Geometry: final body of the model. Coordinates: model frame, mm. A direction names the side the tool comes from. Coordinates: 2 decimals unless noted, no trailing zeros. Order: outer loops, then holes, each group sorted by start corner. A loop starts at its lowest first (then second) coordinate and runs counter-clockwise, first axis right, second up. Notation, with made-up numbers: M 71.25,-22.5 L 75.25,-22.5 A27 ccw 75.25,2.5 Z; hole C 10,89.5 d2. An arc over 180 degrees is marked long. Use CSV: the item, a comma, the result in double quotes. Start each with the question number.
Q1. Section query B-B, the plane y = 0.5. Output: boundary loops of the cut face in (x, z).
Q2. First-contact query: P1, Ø0.5, axis at y = -2.5, z = 1.5, coming from the -X side; P2, Ø2.5, axis at y = -11, z = 3, coming from the -X side; P3, Ø5, axis at x = -29, y = -5, coming from the +Z side. Flat tips, straight axial feed; report the tip coordinate or a pass-through.
Q3. Ray query, probe 1 along Z at (x, y) = (-27, -16.75); probe 2 along X at (y, z) = (2.25, 1.1); probe 3 along X at (y, z) = (-11, 2.65). Return the intervals inside material, ascending.
Q4. Section query A-A, the plane z = 0.4. Output: boundary loops of the cut face in (x, y), and give its area (3 significant figures).
Q5. Section query C-C, the plane x = -43.25. Output: boundary loops of the cut face in (y, z).
Q6. Section query D-D, the plane z = 3.25. Output: boundary loops of the cut face in (x, y).
Q7. Access query for faces 1 (the face through (-31.029, 1.2, 1.5)), 2 (the face through (-33.847, -3.4, 1.5)), 3 (the face through (-38.809, -9, 2)). Directions: +Z, -Z, +X, -X, +Y, -Y. A direction counts if a zero-diameter tool reaches every point of the face in a straight line with its end or side. Return the directions, or none.
Q8. Mould query, pull axis Y, two halves, no side actions, for faces 4 (the face through (-37.259, -3.4, 1.5)), 5 (the face through (-35, -18.555, 0.5)), 6 (the face through (-34.8, 3.625, 1.5)). Classes: +Y half, -Y half, draft (parallel to the pull), parting line (faces both ways), or undercut.
from build123d import *

# Parameters (mm, degrees)
SKETCH1_W               = 25.22
SKETCH1_H               = 23.88
BOSS_EXTRUDE1_DEPTH     = 1
CUT_EXTRUDE1_DEPTH      = 31
CUT_EXTRUDE1_DEPTH_BACK = 15
SKETCH2_R               = 1
BOSS_EXTRUDE2_DEPTH     = 3
SKETCH5_R               = 3.75
BOSS_EXTRUDE4_DEPTH     = 0.74
SKETCH6_R               = 3.4
CUT_EXTRUDE2_DEPTH      = 3
CUT_EXTRUDE3_DEPTH      = 16
CUT_EXTRUDE3_DEPTH_BACK = 20
SKETCH7_R               = 1
BOSS_EXTRUDE5_DEPTH     = 1
SKETCH9_W               = 0.2
SKETCH9_H               = 4.34
CUT_EXTRUDE8_DEPTH      = 1
SKETCH10_W              = 0.124682
SKETCH10_H              = 4.34
CUT_EXTRUDE14_DEPTH     = 1
SKETCH13_W              = 0.120984153
SKETCH13_H              = 4.34
CUT_EXTRUDE15_DEPTH     = 1
SKETCH14_W              = 0.195011185
SKETCH14_H              = 4.311792785
CUT_EXTRUDE18_DEPTH     = 1
SKETCH15_W              = 0.183717696
SKETCH15_H              = 4.326619606
CUT_EXTRUDE21_DEPTH     = 3
SKETCH16_W              = 0.21782098
SKETCH16_H              = 4.34679289
CUT_EXTRUDE22_DEPTH     = 1
SKETCH17_W              = 0.089131755
SKETCH17_H              = 4.34294968
CUT_EXTRUDE23_DEPTH     = 3
SKETCH18_W              = 0.156151398
SKETCH18_H              = 4.341783659
CUT_EXTRUDE24_DEPTH     = 3
SKETCH19_W              = 0.171903048
SKETCH19_H              = 4.300799657
CUT_EXTRUDE26_DEPTH     = 3
SKETCH20_W              = 0.170926161
SKETCH20_H              = 4.327306154
CUT_EXTRUDE28_DEPTH     = 3
SKETCH21_W              = 0.137513245
SKETCH21_H              = 4.32177715
CUT_EXTRUDE29_DEPTH     = 3
SKETCH22_W              = 0.100998317
SKETCH22_H              = 4.324558634
CUT_EXTRUDE30_DEPTH     = 3
SKETCH23_W              = 0.123761921
SKETCH23_H              = 4.331008445
CUT_EXTRUDE31_DEPTH     = 3
SKETCH24_W              = 0.133501637
SKETCH24_H              = 4.354790364
CUT_EXTRUDE32_DEPTH     = 3


with BuildPart() as part:
    # Sketch1 → Boss-Extrude1 (new body)
    with BuildSketch(Plane.XY):
        with Locations((-34.809454486, -6.615438712)):
            Rectangle(SKETCH1_W, SKETCH1_H)
    extrude(amount=BOSS_EXTRUDE1_DEPTH)

    # Sketch2 → Cut-Extrude1 (cut, two sides: drawn at the far end of the back side and taken through both)
    with BuildSketch(Plane.XY.offset(1).offset(-CUT_EXTRUDE1_DEPTH_BACK)):
        with Locations((-24.023789981, 3.500225793)):
            Circle(SKETCH2_R)
        with Locations((-45.59511899, 3.500225793)):
            Circle(SKETCH2_R)
    extrude(amount=CUT_EXTRUDE1_DEPTH + CUT_EXTRUDE1_DEPTH_BACK, mode=Mode.SUBTRACT)

    # Sketch3 → Boss-Extrude2 (add)
    with BuildSketch(Plane.XY.offset(1)):
        Polygon((-34.809454486, -13.555438712), (-30.809454486, -13.555438712), (-30.809454486, -5.555438712), (-38.809454486, -5.555438712), (-38.809454486, -13.555438712), align=None)
    extrude(amount=BOSS_EXTRUDE2_DEPTH)

    # Sketch5 → Boss-Extrude4 (add)
    with BuildSketch(Plane.XY.offset(4)):
        with Locations(Location((-34.860129967, -9.503941157, 0), (0, 0, 180))):
            Circle(SKETCH5_R)
    extrude(amount=BOSS_EXTRUDE4_DEPTH)

    # Sketch6 → Cut-Extrude2 (cut)
    with BuildSketch(Plane.XY.offset(4.74)):
        with Locations((-34.860129967, -9.503941157)):
            Circle(SKETCH6_R)
    extrude(amount=-CUT_EXTRUDE2_DEPTH, mode=Mode.SUBTRACT)

    # Sketch7 → Cut-Extrude3 (cut, two sides: drawn at the far end of the back side and taken through both)
    with BuildSketch(Plane.XY.offset(1).offset(-CUT_EXTRUDE3_DEPTH_BACK)):
        with Locations((-24.023789981, -9.555438712)):
            Circle(SKETCH7_R)
        with Locations((-45.59511899, -9.555438712)):
            Circle(SKETCH7_R)
    extrude(amount=CUT_EXTRUDE3_DEPTH + CUT_EXTRUDE3_DEPTH_BACK, mode=Mode.SUBTRACT)

    # Sketch8 → Boss-Extrude5 (add)
    with BuildSketch(Plane.XY.offset(1)):
        Polygon((-38.589454486, 3.624561288), (-38.589454486, -1.215438712), (-37.609454486, -1.215438712), (-37.609454486, -5.555438712), (-32.009454486, -5.555438712), (-32.009454486, -1.215438712), (-31.029454486, -1.215438712), (-31.029454486, 3.624561288), (-34.809454486, 3.624561288), align=None)
    extrude(amount=BOSS_EXTRUDE5_DEPTH)

    # Sketch9 → Cut-Extrude8 (cut)
    with BuildSketch(Plane.XY.offset(1)):
        with Locations((-37.159454486, -3.385438712)):
            Rectangle(SKETCH9_W, SKETCH9_H)
    extrude(amount=CUT_EXTRUDE8_DEPTH, mode=Mode.SUBTRACT)

    # Sketch10 → Cut-Extrude14 (cut)
    with BuildSketch(Plane.XY.offset(2)):
        with Locations((-36.775157633, -3.385438712)):
            Rectangle(SKETCH10_W, SKETCH10_H)
    extrude(amount=-CUT_EXTRUDE14_DEPTH, mode=Mode.SUBTRACT)

    # Sketch13 → Cut-Extrude15 (cut)
    with BuildSketch(Plane.XY.offset(2)):
        with Locations((-36.400540983, -3.385438712)):
            Rectangle(SKETCH13_W, SKETCH13_H)
    extrude(amount=-CUT_EXTRUDE15_DEPTH, mode=Mode.SUBTRACT)

    # Sketch14 → Cut-Extrude18 (cut)
    with BuildSketch(Plane.XY.offset(1)):
        with Locations((-36.007757653, -3.39954232)):
            Rectangle(SKETCH14_W, SKETCH14_H)
    extrude(amount=CUT_EXTRUDE18_DEPTH, mode=Mode.SUBTRACT)

    # Sketch15 → Cut-Extrude21 (cut)
    with BuildSketch(Plane.XY.offset(4)):
        with Locations((-35.606147547, -3.392128909)):
            Rectangle(SKETCH15_W, SKETCH15_H)
    extrude(amount=-CUT_EXTRUDE21_DEPTH, mode=Mode.SUBTRACT)

    # Sketch16 → Cut-Extrude22 (cut)
    with BuildSketch(Plane.XY.offset(2)):
        with Locations((-35.174485224, -3.382042267)):
            Rectangle(SKETCH16_W, SKETCH16_H)
    extrude(amount=-CUT_EXTRUDE22_DEPTH, mode=Mode.SUBTRACT)

    # Sketch17 → Cut-Extrude23 (cut)
    with BuildSketch(Plane.XY.offset(4)):
        with Locations((-34.764888609, -3.383963872)):
            Rectangle(SKETCH17_W, SKETCH17_H)
    extrude(amount=-CUT_EXTRUDE23_DEPTH, mode=Mode.SUBTRACT)

    # Sketch18 → Cut-Extrude24 (cut)
    with BuildSketch(Plane.XY.offset(4)):
        with Locations((-34.470187586, -3.384546883)):
            Rectangle(SKETCH18_W, SKETCH18_H)
    extrude(amount=-CUT_EXTRUDE24_DEPTH, mode=Mode.SUBTRACT)

    # Sketch19 → Cut-Extrude26 (cut)
    with BuildSketch(Plane.XY.offset(1)):
        with Locations((-34.122346996, -3.405038884)):
            Rectangle(SKETCH19_W, SKETCH19_H)
    extrude(amount=CUT_EXTRUDE26_DEPTH, mode=Mode.SUBTRACT)

    # Sketch20 → Cut-Extrude28 (cut)
    with BuildSketch(Plane.XY.offset(1)):
        with Locations((-33.761764477, -3.391785635)):
            Rectangle(SKETCH20_W, SKETCH20_H)
    extrude(amount=CUT_EXTRUDE28_DEPTH, mode=Mode.SUBTRACT)

    # Sketch21 → Cut-Extrude29 (cut)
    with BuildSketch(Plane.XY.offset(4)):
        with Locations((-33.427485819, -3.394550137)):
            Rectangle(SKETCH21_W, SKETCH21_H)
    extrude(amount=-CUT_EXTRUDE29_DEPTH, mode=Mode.SUBTRACT)

    # Sketch22 → Cut-Extrude30 (cut)
    with BuildSketch(Plane.XY.offset(4)):
        with Locations((-33.108230038, -3.393159395)):
            Rectangle(SKETCH22_W, SKETCH22_H)
    extrude(amount=-CUT_EXTRUDE30_DEPTH, mode=Mode.SUBTRACT)

    # Sketch23 → Cut-Extrude31 (cut)
    with BuildSketch(Plane.XY.offset(4)):
        with Locations((-32.761705251, -3.389934489)):
            Rectangle(SKETCH23_W, SKETCH23_H)
    extrude(amount=-CUT_EXTRUDE31_DEPTH, mode=Mode.SUBTRACT)

    # Sketch24 → Cut-Extrude32 (cut)
    with BuildSketch(Plane.XY.offset(4)):
        with Locations((-32.421390207, -3.37804353)):
            Rectangle(SKETCH24_W, SKETCH24_H)
    extrude(amount=-CUT_EXTRUDE32_DEPTH, mode=Mode.SUBTRACT)


solid = part.part
Responses:
1,outline,"M -47.42,0 L -22.2,0 L -22.2,1 L -31.03,1 L -31.03,2 L -38.59,2 L -38.59,1 L -47.42,1 Z"
2,P1,"stops at x = -37.61"
2,P2,"stops at x = -38.81"
2,P3,"stops at z = 4"
3,probe 1,"z = 0 to 1"
3,probe 2,"x = -38.59 to -31.03"
3,probe 3,"x = -38.81 to -37.91, -31.81 to -30.81"
4,outline,"M -47.42,-18.56 L -22.2,-18.56 L -22.2,5.32 L -47.42,5.32 Z; hole C -45.6,-9.56 d2; hole C -45.6,3.5 d2; hole C -24.02,-9.56 d2; hole C -24.02,3.5 d2"
4,area,"590 mm²"
5,outline,"M -18.56,0 L 5.32,0 L 5.32,1 L -18.56,1 Z"
6,outline,"M -38.81,-13.56 L -30.81,-13.56 L -30.81,-5.56 L -38.81,-5.56 Z; hole C -34.86,-9.5 d6.8"
7,face 1,"+Z, +X, +Y"
7,face 2,"+Z"
7,face 3,"+Z, -X, +Y, -Y"
8,face 4,"undercut"
8,face 5,"-Y half"
8,face 6,"+Y half"
